The listing builds one solid part. Answer for the finished solid, in the listing's coordinates (mm). Coordinates: 2 decimals unless noted, no trailing zeros. Loops run counter-clockwise (first coordinate to the right, second up) from the corner with the lowest first, then second, coordinate; pieces in that order, holes last. Notation, with made-up numbers: (54.5, -26.75) - (91.5, -26.75) arc R9 ccw to (91.5, -16.75) - close; hole circle Ø5 at (10, 43). An arc over 180 degrees is marked (long way). Use one line per item in the form item = value. Start each with the question number.
Autodesk Inventor part; units mm, degrees
ref_plane "YZ Plane" through (0, 0, 0) normal (1, 0, 0) x (0, 1, 0)
ref_plane "XZ Plane" through (0, 0, 0) normal (0, 1, 0) x (-1, 0, 0)
ref_plane "XY Plane" through (0, 0, 0) normal (0, 0, 1) x (1, 0, 0)
sketch "Sketch1" plane through (0, 0, 0) normal (0, 1, 0) x (-1, 0, 0)
  circle A0 centre (0, 0) radius 15
  circle A1 centre (0, 0) radius 92.5 construction
  line L0 (115, -37.3658) -> (71.0739, -97.8248) construction
  line L1 (71.0739, -97.8248) -> (0, -120.9182) construction
  line L2 (0, -120.9182) -> (-71.0739, -97.8248) construction
  line L3 (-71.0739, -97.8248) -> (-115, -37.3658) construction
  line L4 (-115, -37.3658) -> (-115, 37.3658) construction
  line L5 (-115, 37.3658) -> (-71.0739, 97.8248) construction
  line L6 (-71.0739, 97.8248) -> (0, 120.9182) construction
  line L7 (0, 120.9182) -> (71.0739, 97.8248) construction
  line L8 (71.0739, 97.8248) -> (115, 37.3658) construction
  line L9 (115, 37.3658) -> (115, -37.3658) construction
  line L10 (0, 0) -> (0, -190.4975) construction
  line L11 (45.6611, -109.9595) -> (-45.4658, -110.0404)
  line L12 (-45.4658, -110.0404) -> (-109.9595, -45.6611)
  line L13 (-109.9595, -45.6611) -> (-110.0404, 45.4658)
  line L14 (-110.0404, 45.4658) -> (-45.6611, 109.9595)
  line L15 (-45.6611, 109.9595) -> (45.4658, 110.0404)
  line L16 (45.4658, 110.0404) -> (109.9595, 45.6611)
  line L17 (109.9595, 45.6611) -> (110.0404, -45.4658)
  line L18 (110.0404, -45.4658) -> (45.6611, -109.9595)
  dimension "d0" = 30
  dimension "d1" = 185
  dimension "d4" = 230
  dimension "d18" = 220
extrude "Extrusion1" add sketch "Sketch1" along normal blind 5
sketch "Sketch2" plane through (0, 5, 0) normal (0, 1, 0) x (1, 0, 0)
  line L0 (0, 0) -> (-95, 0) construction
  line L1 (-106.25, -6.75) -> (-83.75, -6.75) construction
  line L2 (-83.75, -6.75) -> (-83.75, 6.75) construction
  line L3 (-83.75, 6.75) -> (-106.25, 6.75) construction
  line L4 (-106.25, 6.75) -> (-106.25, -6.75) construction
  line L5 (-106.25, -6.75) -> (-83.75, 6.75) construction
  line L6 (-83.75, -6.75) -> (-106.25, 6.75) construction
  circle A0 centre (-106.25, -6.75) radius 1
  circle A1 centre (-106.25, 6.75) radius 1
  circle A2 centre (-83.75, 6.75) radius 1
  circle A3 centre (-83.75, -6.75) radius 1
  line L7 (-115, 37.3658) -> (-115, -37.3658)
  line L8 (-110.0404, 45.4658) -> (-109.9595, -45.6611)
  dimension "d5" = 22.5
  dimension "d6" = 13.5
  dimension "d7" = 2
  dimension "d8" = 2
  dimension "d9" = 2
  dimension "d10" = 2
  dimension "d19" = 15
extrude "Extrusion2" cut sketch "Sketch2" against normal blind 5
pattern_circular "Circular Pattern1" count 8 over 360 about axis through (0, 0, 0) along (0, 1, 0) of "Extrusion2"
fillet "Fillet1" radius 10 8 edges at (-45.4658, 2.5, 110.0404) (45.6611, 2.5, 109.9595) (110.0404, 2.5, 45.4658) (109.9595, 2.5, -45.6611) (45.4658, 2.5, -110.0404) (-45.6611, 2.5, -109.9595) (-110.0404, 2.5, -45.4658) (-109.9595, 2.5, 45.6611)
sketch "Sketch3" plane through (0, 5, 0) normal (0, 1, 0) x (1, 0, 0)
  circle A0 centre (-99.9734, -30) radius 1.5 construction
  line L0 (-110.0367, 41.3237) -> (-109.9632, -41.519)
  line L1 (0, 0) -> (-110, -0.0977)
  line L2 (0, 0) -> (-110, -0.0977)
  line L3 (-110, -0.0977) -> (-134, -0.0977) construction
  circle A1 centre (-99.9734, 29.8047) radius 1.5 construction
  arc A2 (-109.9632, -41.519) -> (-107.028, -48.5875) centre (-99.9632, -41.5101) ccw
  line L4 (0, 0) -> (-99.9632, -41.5101) construction
  line L5 (-99.9632, -41.5101) -> (-109.1986, -45.3452) construction
  circle A3 centre (-102, -42.3559) radius 1.55
  dimension "d22" = 3
  dimension "d23" = 30
  dimension "d24" = 10
  dimension "d30" = 3.1
  dimension "d31" = 102
extrude "Extrusion3" cut sketch "Sketch3" against normal blind 10
pattern_circular "Circular Pattern2" count 8 over 360 about axis through (0, 0, 0) along (0, 1, 0) of "Extrusion3"
sketch "Sketch4" plane through (0, 5, 0) normal (0, 1, 0) x (1, 0, 0)
  line L0 (-50, 0) -> (50, 0)
  line L1 (50, 0) -> (50, -118)
  line L2 (50, -118) -> (-50, -118)
  line L3 (-50, -118) -> (-50, 0)
  point P0 (0, 0)
  dimension "d32" = 50
  dimension "d33" = 50
  dimension "d34" = 118
extrude "Extrusion4" cut sketch "Sketch4" against normal blind 10 keep common part
sketch "Sketch5" plane through (0, 5, 0) normal (0, 1, 0) x (1, 0, 0)
  circle A0 centre (-37.5, -90.0333) radius 3
  line L0 (-50, -105.5143) -> (-50, 0)
  line L1 (-41.3237, -110.0367) -> (41.519, -109.9632)
  point P0 (0, 0)
  dimension "d37" = 6
  dimension "d38" = 12.5
  dimension "d39" = 20
extrude "Extrusion5" cut sketch "Sketch5" against normal blind 10
pattern_linear "Rectangular Pattern1" count 4 spacing 25 along (0, 0, -1) count 4 spacing 25 along (1, 0, -0.0009) of "Extrusion5"
sketch "Sketch6" plane through (0, 5, 0) normal (0, 1, 0) x (1, 0, 0)
  circle A0 centre (-3.25, -19.25) radius 1
  circle A1 centre (-6.75, -83.75) radius 1
  line L0 (0, 0) -> (0, -32) construction
  circle A2 centre (3.25, -19.25) radius 1
  dimension "d48" = 2
  dimension "d49" = 64.5
  dimension "d50" = 3.5
extrude "Extrusion6" cut sketch "Sketch6" against normal blind 10 contours A0 | A2
properties part number "Base"
(1) Find the intervals of material crossed by probe 1 along Z at (x, y) = (-6.75, 2.7); probe 2 along X at (y, z) = (3.2, 106.25); probe 3 along Z at (x, y) = (-35.5, 4.65), in increasing order. Write a range as from..to.
(2) Determine the mould class of faces 1 (the face through (1, 5, 56)), 2 (the face through (32, 3, 0)), 3 (the face through (36.85, 2.535, 67.894)) for opening direction Z: +Z half, -Z half, draft (parallel to the pull), parting line (faces both ways), or undercut.
(3) Each of these flat-tipped pins is pushed along its axis until it touches: pin 1 Ø2.5 at (x, z) = (-6.75, 83.75) entering from -Y; pin 2 Ø3 at (x, y) = (7.5, 0.5) entering from +Z. Where does it stop, or does it pass through?
(4) A cutting plane is placed at C-C (x = -0.5). Determine the outline of the cut face in (y, z).
(5) A cutting plane is placed at B-B (y = 2.3). State how many separate pieces and enclosed holes the cut face has, then the cut area to 3 significant figures.
(6) A cutting plane is placed at A-A (x = -37.5). Determine the outline of the cut face in (y, z), then the cut area to 3 significant figures.
Evaluation:
q1.probe_1 = 13.4..82.75, 84.75..105.25, 107.25..110.01
q1.probe_2 = -49.26..-7.75, -5.75..5.75, 7.75..49.36
q1.probe_3 = 0..12.8, 17.27..37.8, 42.27..62.8, 67.27..87.8, 92.27..110.03
q2.face_1 = draft
q2.face_2 = -Z half
q2.face_3 = undercut
q3.pin_1 = 0
q3.pin_2 = 109.99
q4.outline = (0, 14.99) - (5, 14.99) - (5, 110) - (0, 110) - close
q5.separate_pieces = 1
q5.enclosed_holes = 24
q5.area = 10,100 mm^2
q6.outline = (0, 0) - (5, 0) - (5, 12.03) - (0, 12.03) - close; (0, 18.03) - (5, 18.03) - (5, 37.03) - (0, 37.03) - close; (0, 43.03) - (5, 43.03) - (5, 62.03) - (0, 62.03) - close; (0, 68.03) - (5, 68.03) - (5, 87.03) - (0, 87.03) - close; (0, 93.03) - (5, 93.03) - (5, 110.03) - (0, 110.03) - close
q6.area = 430 mm^2
